Design review of the part built by this model. Coordinates are the model's own, in mm. Round coordinates to 2 decimals unless told otherwise and drop trailing zeros.
Autodesk Inventor part; units mm, degrees
ref_plane "YZ Plane" through (0, 0, 0) normal (1, 0, 0) x (0, 1, 0)
ref_plane "XZ Plane" through (0, 0, 0) normal (0, 1, 0) x (-1, 0, 0)
ref_plane "XY Plane" through (0, 0, 0) normal (0, 0, 1) x (1, 0, 0)
sketch "Skin Scheme" plane through (0, 0, 0) normal (0, 1, 0) x (-1, 0, 0)
  line L0 (835, -84.5) -> (-835, -84.5)
  line L1 (-835, -84.5) -> (-835, 84.5)
  line L2 (-835, 84.5) -> (835, 84.5)
  line L3 (835, 84.5) -> (835, -84.5)
  circle A0 centre (713, -62.5) radius 5
  circle A1 centre (667, -62.5) radius 5
  circle A2 centre (621, -62.5) radius 5
  circle A3 centre (575, -62.5) radius 5
  circle A4 centre (529, -62.5) radius 5
  circle A5 centre (483, -62.5) radius 5
  circle A6 centre (437, -62.5) radius 5
  circle A7 centre (391, -62.5) radius 5
  circle A8 centre (345, -62.5) radius 5
  circle A9 centre (299, -62.5) radius 5
  circle A10 centre (253, -62.5) radius 5
  circle A11 centre (207, -62.5) radius 5
  circle A12 centre (161, -62.5) radius 5
  circle A13 centre (115, -62.5) radius 5
  circle A14 centre (69, -62.5) radius 5
  circle A15 centre (23, -62.5) radius 5
  circle A16 centre (-23, -62.5) radius 5
  circle A17 centre (-69, -62.5) radius 5
  circle A18 centre (713, 62.5) radius 5
  circle A19 centre (667, 62.5) radius 5
  circle A20 centre (621, 62.5) radius 5
  circle A21 centre (575, 62.5) radius 5
  circle A22 centre (529, 62.5) radius 5
  circle A23 centre (483, 62.5) radius 5
  circle A24 centre (437, 62.5) radius 5
  circle A25 centre (391, 62.5) radius 5
  circle A26 centre (345, 62.5) radius 5
  circle A27 centre (299, 62.5) radius 5
  circle A28 centre (253, 62.5) radius 5
  circle A29 centre (207, 62.5) radius 5
  circle A30 centre (161, 62.5) radius 5
  circle A31 centre (115, 62.5) radius 5
  circle A32 centre (69, 62.5) radius 5
  circle A33 centre (23, 62.5) radius 5
  circle A34 centre (-23, 62.5) radius 5
  circle A35 centre (-69, 62.5) radius 5
  circle A36 centre (-115, -62.5) radius 5
  circle A37 centre (-115, 62.5) radius 5
  circle A38 centre (-161, -62.5) radius 5
  circle A39 centre (-161, 62.5) radius 5
  circle A40 centre (-207, -62.5) radius 5
  circle A41 centre (-207, 62.5) radius 5
  circle A42 centre (-253, -62.5) radius 5
  circle A43 centre (-253, 62.5) radius 5
  circle A44 centre (-299, -62.5) radius 5
  circle A45 centre (-299, 62.5) radius 5
  circle A46 centre (-345, -62.5) radius 5
  circle A47 centre (-345, 62.5) radius 5
  circle A48 centre (-391, -62.5) radius 5
  circle A49 centre (-391, 62.5) radius 5
  circle A50 centre (-437, -62.5) radius 5
  circle A51 centre (-437, 62.5) radius 5
  circle A52 centre (-483, -62.5) radius 5
  circle A53 centre (-483, 62.5) radius 5
  circle A54 centre (-529, -62.5) radius 5
  circle A55 centre (-529, 62.5) radius 5
  circle A56 centre (-575, -62.5) radius 5
  circle A57 centre (-575, 62.5) radius 5
  circle A58 centre (-621, -62.5) radius 5
  circle A59 centre (-621, 62.5) radius 5
  circle A60 centre (-667, -62.5) radius 5
  circle A61 centre (-667, 62.5) radius 5
  circle A62 centre (-713, -62.5) radius 5
  circle A63 centre (-713, 62.5) radius 5
  point P0 (0, 0)
  dimension "d0" = 1670
  dimension "d1" = 835
  dimension "d2" = 169
  dimension "d3" = 84.5
  dimension "d4" = 10
  dimension "d5" = 122
  dimension "d6" = 22
  dimension "d9" = 46
  dimension "d12" = 125
extrude "Skin Body" add sketch "Skin Scheme" along normal blind 1
sketch "End Cut Outline" plane through (0, 1, 0) normal (0, 1, 0) x (1, 0, 0)
  line L0 (-785, 94.5) -> (-845, 94.5)
  line L1 (-845, 94.5) -> (-845, -94.5)
  line L2 (-845, -94.5) -> (-785, -94.5)
  line L3 (-785, -94.5) -> (-785, 94.5)
  line L4 (835, 84.5) -> (-835, 84.5)
  line L5 (-835, -84.5) -> (835, -84.5)
  line L6 (-835, 84.5) -> (-835, -84.5)
  point P0 (0, 0)
  dimension "d19" = 10
  dimension "d20" = 10
  dimension "d21" = 10
  dimension "d22" = 50
extrude "End Cut" cut sketch "End Cut Outline" along normal through all both and the other way through all
mirror "End Cut Mirror" about plane through (0, 0, 0) normal (1, 0, 0) of "End Cut"
properties part number "Skin NPS 16 Internal" material "Rubber, Silicone"
1) For line 1 along Z through (x, y) = (713, 0.3); line 2 along Z through (x, y) = (-530.5, 0.9), list the stretches that pass through material, from the lowest coordinate up.
2) For P1, Ø16, axis at x = 207, z = -62.5, coming from the -Y side, flat-tipped, find the tip position at first contact; note if it passes through.
3) Add section A-A on y = 0.7. Count the separate pieces of the cut face and the enclosed holes in it, and give its area (3 significant figures).
Computed:
1. line 1: z = -84.5 to -67.5, -57.5 to 57.5, 67.5 to 84.5
1. line 2: z = -84.5 to -67.27, -57.73 to 57.73, 67.27 to 84.5
2. P1: stops at y = 0
3. separate pieces: 1
3. enclosed holes: 64
3. area: 260,000 mm2
